from build123d import *

# Parameters (mm, degrees)
F0_R     = 63.5
F1_DEPTH = 25.4
F2_R     = 76.2
F3_DEPTH = 25.4


with BuildPart() as f1:
    # F0 (on Front) → F1 (new body)
    with BuildSketch(Plane.XZ):
        Circle(F0_R)
    extrude(amount=F1_DEPTH)


with BuildPart() as f3:
    # F2 (on Top) → F3 (new body)
    with BuildSketch(Plane.XY):
        with Locations((-51.968064, -67.365818)):
            Circle(F2_R)
    extrude(amount=F3_DEPTH)


with BuildPart() as f1_1:
    add(f1.part)

    # F4: cut F3
    add(f3.part, mode=Mode.SUBTRACT)


solid = f1_1.part
Design review of the part built by this model. Coordinates are the model's own, in mm. A direction names the side the tool comes from. Give positions to 0.01 mm unless a question says otherwise; leave off trailing zeros. Order: outer loops, then holes, each group sorted by start corner. A loop starts at its lowest first (then second) coordinate and runs counter-clockwise, first axis right, second up.
1. Add section B-B, the plane x = 0. State the section outline as (y, z) points, then the cut area to 3 significant figures.
Solution:
outline: (-25.4, -63.5) - (0, -63.5) - (0, 63.5) - (-25.4, 63.5) - (-25.4, 25.4) - (-11.64, 25.4) - (-11.64, 0) - (-25.4, 0) - close
area: 2,880 mm2
2. To check wall thickness, follow L1, parallel to Z at x = -22, y = -5.5; L2, parallel to Z at x = -21.5, y = -23; L3, parallel to Z at x = -2, y = -9.5. State the ranges of each line that lie inside material, in increasing order.
Solution:
L1: z = -59.57 to 0, 25.4 to 59.57
L2: z = -59.75 to 0, 25.4 to 59.75
L3: z = -63.47 to 63.47
3. Add section C-C, the plane y = -20. State the section outline as (x, z) points.
Solution:
outline: (-63.5, 0) arc R63.5 ccw (long way) to (-58.2, 25.4) - (7.72, 25.4) - (7.72, 0) - close
4. Mouldability with a two-part tool opening along Z and no side actions: class faces 3 (the flat face through (-32, -13, 25.4)), 4 (the cylindrical face through (-0.56, -11.12, 12.52)), 5 (the cylindrical face through (61.575, -12.522, -15.517)), 6 (the flat face through (13, -25.4, 1)) as +Z half, -Z half, draft (parallel to the pull), parting line (faces both ways), or undercut.
Solution:
face 3: undercut
face 4: undercut
face 5: parting line
face 6: draft
5. For pin 1 Ø5 at (x, y) = (39, -9) entering from +Z; pin 2 Ø10 at (x, y) = (-32.5, -4) entering from +Z; pin 3 Ø3 at (x, y) = (-46.5, -20.5) entering from -Z, all flat-tipped, find the tip position at first contact; note any pin that passes through.
Solution:
pin 1: stops at z = 51.96
pin 2: stops at z = 57.24
pin 3: stops at z = -44.8
6. Tool access review of faces 1 (the flat face through (-1, 0, 1)), 2 (the flat face through (-35, -13, 0)): name each direction out of +Z, -Z, +X, -X, +Y, -Y from which nothing blocks a thin tool from reaching the whole face with its end or side.
Solution:
face 1: +Z, -Z, +X, -X, +Y
face 2: -X, -Y
7. Add section A-A, the plane x = -33.5. State the section outline as (y, z) points, then the cut area to 3 significant figures.
Solution:
outline: (-25.4, -53.94) - (0, -53.94) - (0, 0) - (-25.4, 0) - close; (-25.4, 25.4) - (0, 25.4) - (0, 53.94) - (-25.4, 53.94) - close
area: 2,100 mm2
8. Add section D-D, the plane z = 35.5. State the section outline as (x, y) points.
Solution:
outline: (-52.65, -25.4) - (52.65, -25.4) - (52.65, 0) - (-52.65, 0) - close
